Read the model definition and answer for the solid it produces. Units are mm, in the model's axes. Face numbers are marked on the shaded views. A direction names the side the tool comes from. Coordinates: 2 decimals unless noted, no trailing zeros. Write each loop counter-clockwise with the first axis right and the second up, starting at its lowest first coordinate (ties: lowest second). Pieces come first, ordered by that corner, then holes. Notation, with made-up numbers: (8, 43) -> (66, 43) arc R26 ccw to (66, 66) -> close; hole circle Ø5 at (-12, 46.5). An arc over 180 degrees is marked (long way). Write item = value, one per line. Start each with the question number.
1) A tool of negligible diameter and unlimited length cuts with its end or side. For the marked faces 1, 2, 3, 4 and 5, from which of +Z, -Z, +X, -X, +Y, -Y can it reach the whole face along a straight path? Write none if from no direction.
2) Section A-A (y = 0) is taken. Determine the outline of the cut face in (x, z).
3) Section B-B (z = -18) is taken. Determine the outline of the cut face in (x, y), plus the area to 3 significant figures.
4) Find the intervals of material crossed by line 1 along Z through (x, y) = (0, -0.5); line 2 along Y through (x, z) = (-7, 0); line 3 along Z through (x, y) = (-7.1, 0), in increasing order. Write a range as from..to.
5) For a pull along X with two mould halves and no side action, classify the marked faces 6, 7 and 8 as released by +X, released by -X, zero draft, split by the parting line, or undercut.
6) Section D-D (x = -1) is taken. Count the separate pieces of the cut face and the enclosed holes in it, plus the area to 3 significant figures.
7) Section C-C (z = -4) is taken. Determine the outline of the cut face in (x, y).
8) Flat-ended cylindrical pins translate along their axes: pin 1 Ø19 at (x, z) = (0, -18) entering from -Y; pin 2 Ø5 at (y, z) = (0, 0) entering from +X; pin 3 Ø3.5 at (y, z) = (0, -18) entering from -X; pin 4 Ø3 at (x, y) = (-1.5, -3) entering from +Z. Find the tip coordinate at first contact, or state that the pin passes through.
from build123d import *
from OCP.BRepFilletAPI import BRepFilletAPI_MakeChamfer

# Parameters (mm, degrees)
BOSS_EXTRUDE1_DEPTH     = 5
FILLET1_R               = 4
SKETCH2_R               = 8
BOSS_EXTRUDE2_DEPTH     = 0.5
SKETCH3_R               = 8
BOSS_EXTRUDE3_DEPTH     = 0.5
SKETCH4_R               = 8
BOSS_EXTRUDE4_DEPTH     = 0.5
CUT_EXTRUDE1_DEPTH      = 43.969085178
CUT_EXTRUDE1_DEPTH_BACK = 43.969085178
SKETCH5_R               = 6
CUT_EXTRUDE2_DEPTH      = 2
CHAMFER2_SIZE           = 1
CHAMFER2_SIZE2          = 1.732050808
CUT_EXTRUDE4_DEPTH      = 42.899788694
CUT_EXTRUDE4_DEPTH_BACK = 42.899788694
SKETCH9_R               = 1.5


with BuildPart() as part:
    # Sketch1 → Boss-Extrude1 (new, symmetric)
    with BuildSketch(Plane(origin=(0, 0, 0), x_dir=(1, 0, 0), z_dir=(0, 1, 0))):
        with BuildLine():
            Line((-10, 30.489995997), (-10, -2.679491924))
            Line((-10, -2.679491924), (-25.114071484, -6.729295173))
            ThreePointArc((-25.114071484, -6.729295173), (0, -26), (25.114071484, -6.729295173))
            Line((25.114071484, -6.729295173), (10, -2.679491924))
            Line((10, -2.679491924), (10, 30.489995997))
            ThreePointArc((10, 30.489995997), (0, 34), (-10, 30.489995997))
        make_face()
    extrude(amount=BOSS_EXTRUDE1_DEPTH, both=True)

    # Fillet1
    fillet1_edges = [part.edges().sort_by_distance(p)[0] for p in [
        (10, 0, -30.489995997),
        (10, 0, 2.679491924),
        (25.114071484, 0, 6.729295173),
        (-25.114071484, 0, 6.729295173),
        (-10, 0, 2.679491924),
        (-10, 0, -30.489995997),
    ]]
    fillet(fillet1_edges, radius=FILLET1_R)

    # Sketch2 → Boss-Extrude2 (add, symmetric)
    with BuildSketch(Plane(origin=(0, 0, 0), x_dir=(1, 0, 0), z_dir=(0, 1, 0))):
        with Locations((0, 18)):
            Circle(SKETCH2_R)
    extrude(amount=BOSS_EXTRUDE2_DEPTH, both=True)

    # Sketch3 → Boss-Extrude3 (add, symmetric)
    with BuildSketch(Plane(origin=(0, 5, 0), x_dir=(1, 0, 0), z_dir=(0, 1, 0))):
        with Locations(Location((0, 18, 0), (0, 0, 270))):
            Circle(SKETCH3_R)
    extrude(amount=BOSS_EXTRUDE3_DEPTH, both=True)

    # Sketch4 → Boss-Extrude4 (add, symmetric)
    with BuildSketch(Plane.XZ.offset(5)):
        with Locations(Location((0, 0, 0), (0, 0, 90))):
            Circle(SKETCH4_R)
    extrude(amount=BOSS_EXTRUDE4_DEPTH, both=True)

    # Sketch5 → Cut-Extrude1 (cut, two sides: drawn at the far end of the back side and taken through both)
    with BuildSketch(Plane(origin=(0, -5.5, 0), x_dir=(-1, 0, 0), z_dir=(0, -1, 0)).offset(-CUT_EXTRUDE1_DEPTH_BACK)):
        with Locations(Location((0, 0, 0), (0, 0, 90))):
            Circle(SKETCH5_R)
        with Locations(Location((0, 18, 0), (0, 0, 90))):
            Circle(SKETCH5_R)
    extrude(amount=CUT_EXTRUDE1_DEPTH + CUT_EXTRUDE1_DEPTH_BACK, mode=Mode.SUBTRACT)

    # Sketch6 → Cut-Extrude2 (cut)
    with BuildSketch(Plane(origin=(0, 5, 0), x_dir=(1, 0, 0), z_dir=(0, 1, 0))):
        with BuildLine():
            Line((12.188266684, -6.371664756), (20.119713435, -8.496889508))
            ThreePointArc((20.119713435, -8.496889508), (20.768948696, -9.043962883), (20.763662316, -9.892943304))
            ThreePointArc((20.763662316, -9.892943304), (0, -23), (-20.763662316, -9.892943304))
            ThreePointArc((-20.763662316, -9.892943304), (-20.768948696, -9.043962883), (-20.119713435, -8.496889508))
            Line((-20.119713435, -8.496889508), (-12.188266684, -6.371664756))
            ThreePointArc((-12.188266684, -6.371664756), (-11.342355786, -6.086056673), (-10.539679728, -5.695098402))
            ThreePointArc((-10.539679728, -5.695098402), (-9.810114884, -5.592432974), (-9.208235905, -6.017340901))
            ThreePointArc((-9.208235905, -6.017340901), (0, -11), (9.208235905, -6.017340901))
            ThreePointArc((9.208235905, -6.017340901), (9.810114884, -5.592432974), (10.539679728, -5.695098402))
            ThreePointArc((10.539679728, -5.695098402), (11.342355786, -6.086056673), (12.188266684, -6.371664756))
        make_face()
    cut_extrude2 = extrude(amount=-CUT_EXTRUDE2_DEPTH, mode=Mode.SUBTRACT)

    # Mirror7: Cut-Extrude2 across plane
    add(cut_extrude2.mirror(Plane.ZX), mode=Mode.SUBTRACT)

    # Chamfer2: one chamfer whose edges measure the first distance from different faces: ONE call of the kernel's chamfer builder (chamfer() names one face for all edges)
    chamfer2_edges_1 = [part.edges().sort_by_distance(p)[0] for p in [
        (9.810114884, -5, 5.592432974),
        (0, -5, 11),
        (-9.810114884, -5, 5.592432974),
        (-11.342355786, -5, 6.086056673),
        (-16.153990059, -5, 7.434277132),
        (-20.768948696, -5, 9.043962883),
        (0, -5, 23),
        (20.768948696, -5, 9.043962883),
        (16.153990059, -5, 7.434277132),
        (11.342355786, -5, 6.086056673),
    ]]
    chamfer2_side_1 = [part.faces().sort_by_distance(p)[0] for p in [
        (-9.233359985, -5, -14.391060437),
    ]]
    chamfer2_edges_2 = [part.edges().sort_by_distance(p)[0] for p in [
        (9.810114884, 5, 5.592432974),
    ]]
    chamfer2_side_2 = [part.faces().sort_by_distance(p)[0] for p in [
        (9.810114884, 4, 5.592432974),
    ]]
    chamfer2_edges_3 = [part.edges().sort_by_distance(p)[0] for p in [
        (0, 5, 11),
    ]]
    chamfer2_side_3 = [part.faces().sort_by_distance(p)[0] for p in [
        (0, 4, 11),
    ]]
    chamfer2_edges_4 = [part.edges().sort_by_distance(p)[0] for p in [
        (-9.810114884, 5, 5.592432974),
    ]]
    chamfer2_side_4 = [part.faces().sort_by_distance(p)[0] for p in [
        (-9.810114884, 4, 5.592432974),
    ]]
    chamfer2_edges_5 = [part.edges().sort_by_distance(p)[0] for p in [
        (-11.342355786, 5, 6.086056673),
    ]]
    chamfer2_side_5 = [part.faces().sort_by_distance(p)[0] for p in [
        (-11.342355786, 4, 6.086056673),
    ]]
    chamfer2_edges_6 = [part.edges().sort_by_distance(p)[0] for p in [
        (-16.153990059, 5, 7.434277132),
    ]]
    chamfer2_side_6 = [part.faces().sort_by_distance(p)[0] for p in [
        (-16.153990059, 4, 7.434277132),
    ]]
    chamfer2_edges_7 = [part.edges().sort_by_distance(p)[0] for p in [
        (-20.768948696, 5, 9.043962883),
    ]]
    chamfer2_side_7 = [part.faces().sort_by_distance(p)[0] for p in [
        (-20.768948696, 4, 9.043962883),
    ]]
    chamfer2_edges_8 = [part.edges().sort_by_distance(p)[0] for p in [
        (0, 5, 23),
    ]]
    chamfer2_side_8 = [part.faces().sort_by_distance(p)[0] for p in [
        (0, 4, 23),
    ]]
    chamfer2_edges_9 = [part.edges().sort_by_distance(p)[0] for p in [
        (20.768948696, 5, 9.043962883),
    ]]
    chamfer2_side_9 = [part.faces().sort_by_distance(p)[0] for p in [
        (20.768948696, 4, 9.043962883),
    ]]
    chamfer2_edges_10 = [part.edges().sort_by_distance(p)[0] for p in [
        (16.153990059, 5, 7.434277132),
    ]]
    chamfer2_side_10 = [part.faces().sort_by_distance(p)[0] for p in [
        (16.153990059, 4, 7.434277132),
    ]]
    chamfer2_edges_11 = [part.edges().sort_by_distance(p)[0] for p in [
        (11.342355786, 5, 6.086056673),
    ]]
    chamfer2_side_11 = [part.faces().sort_by_distance(p)[0] for p in [
        (11.342355786, 4, 6.086056673),
    ]]
    chamfer2 = BRepFilletAPI_MakeChamfer(part.part.solid().wrapped)
    for e in chamfer2_edges_1:
        chamfer2.Add(CHAMFER2_SIZE, CHAMFER2_SIZE2, e.wrapped, chamfer2_side_1[0].wrapped)  # the first distance lies on this face
    for e in chamfer2_edges_2:
        chamfer2.Add(CHAMFER2_SIZE, CHAMFER2_SIZE2, e.wrapped, chamfer2_side_2[0].wrapped)  # the first distance lies on this face
    for e in chamfer2_edges_3:
        chamfer2.Add(CHAMFER2_SIZE, CHAMFER2_SIZE2, e.wrapped, chamfer2_side_3[0].wrapped)  # the first distance lies on this face
    for e in chamfer2_edges_4:
        chamfer2.Add(CHAMFER2_SIZE, CHAMFER2_SIZE2, e.wrapped, chamfer2_side_4[0].wrapped)  # the first distance lies on this face
    for e in chamfer2_edges_5:
        chamfer2.Add(CHAMFER2_SIZE, CHAMFER2_SIZE2, e.wrapped, chamfer2_side_5[0].wrapped)  # the first distance lies on this face
    for e in chamfer2_edges_6:
        chamfer2.Add(CHAMFER2_SIZE, CHAMFER2_SIZE2, e.wrapped, chamfer2_side_6[0].wrapped)  # the first distance lies on this face
    for e in chamfer2_edges_7:
        chamfer2.Add(CHAMFER2_SIZE, CHAMFER2_SIZE2, e.wrapped, chamfer2_side_7[0].wrapped)  # the first distance lies on this face
    for e in chamfer2_edges_8:
        chamfer2.Add(CHAMFER2_SIZE, CHAMFER2_SIZE2, e.wrapped, chamfer2_side_8[0].wrapped)  # the first distance lies on this face
    for e in chamfer2_edges_9:
        chamfer2.Add(CHAMFER2_SIZE, CHAMFER2_SIZE2, e.wrapped, chamfer2_side_9[0].wrapped)  # the first distance lies on this face
    for e in chamfer2_edges_10:
        chamfer2.Add(CHAMFER2_SIZE, CHAMFER2_SIZE2, e.wrapped, chamfer2_side_10[0].wrapped)  # the first distance lies on this face
    for e in chamfer2_edges_11:
        chamfer2.Add(CHAMFER2_SIZE, CHAMFER2_SIZE2, e.wrapped, chamfer2_side_11[0].wrapped)  # the first distance lies on this face
    add(Compound.cast(chamfer2.Shape()), mode=Mode.REPLACE)

    # Sketch9 → Cut-Extrude4 (cut, two sides: drawn at the far end of the back side and taken through both)
    with BuildSketch(Plane(origin=(0, 0, 0), x_dir=(0, 0, -1), z_dir=(1, 0, 0)).offset(-CUT_EXTRUDE4_DEPTH_BACK)):
        Circle(SKETCH9_R)
        with Locations((18, 0)):
            Circle(SKETCH9_R)
    extrude(amount=CUT_EXTRUDE4_DEPTH + CUT_EXTRUDE4_DEPTH_BACK, mode=Mode.SUBTRACT)


solid = part.part
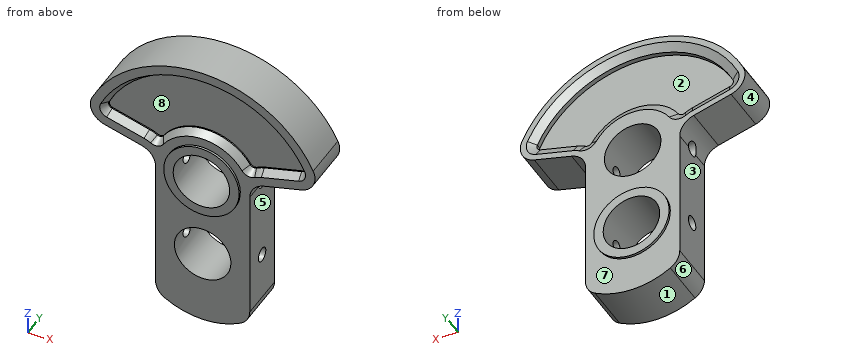
Answer key:
q1.face_1 = -Z, +Y, -Y
q1.face_2 = +Y
q1.face_3 = -Z, -X, +Y, -Y
q1.face_4 = -X, +Y, -Y
q1.face_5 = -Z, +X, +Y, -Y
q2.outline = (-23.47, 11.18) arc R4 ccw to (-20.9, 5.6) -> (-12.96, 3.47) arc R4 cw to (-10.47, 1.5) -> (-5.81, 1.5) arc R6 cw to (5.81, 1.5) -> (10.47, 1.5) arc R4 cw to (12.96, 3.47) -> (20.9, 5.6) arc R4 ccw to (23.47, 11.18) arc R26 ccw to start; (-10, -28.39) arc R4 ccw to (-8, -31.86) arc R16 ccw to (8, -31.86) arc R4 ccw to (10, -28.39) -> (10, -19.5) -> (5.81, -19.5) arc R6 cw to (-5.81, -19.5) -> (-10, -19.5) -> close; (-10, -16.5) -> (-5.81, -16.5) arc R6 cw to (5.81, -16.5) -> (10, -16.5) -> (10, -1.5) -> (5.81, -1.5) arc R6 cw to (-5.81, -1.5) -> (-10, -1.5) -> close
q3.outline = (-10, -5) -> (-6, -5) -> (-6, -1.5) -> (-10, -1.5) -> close; (-10, 1.5) -> (-6, 1.5) -> (-6, 5.5) -> (-8, 5.5) -> (-8, 5) -> (-10, 5) -> close; (6, -5) -> (10, -5) -> (10, -1.5) -> (6, -1.5) -> close; (6, 1.5) -> (10, 1.5) -> (10, 5) -> (8, 5) -> (8, 5.5) -> (6, 5.5) -> close
q3.area = 58.0 mm^2
q4.line_1 = -34..-24, -12..-6, 6..26
q4.line_2 = -5.5..-1.5, 1.5..5
q4.line_3 = -32.34..-19.5, -16.5..-1.5, 1.5..25.01
q5.face_6 = released by -X
q5.face_7 = zero draft
q5.face_8 = undercut
q6.separate_pieces = 3
q6.enclosed_holes = 0
q6.area = 315 mm^2
q7.outline = (-10, -5) -> (-6.93, -5) -> (-6.93, -5.5) -> (-4.47, -5.5) -> (-4.47, 5) -> (-10, 5) -> close; (4.47, -5.5) -> (6.93, -5.5) -> (6.93, -5) -> (10, -5) -> (10, 5) -> (4.47, 5) -> close
q8.pin_1 = -5
q8.pin_2 = 11.23
q8.pin_3 = -10
q8.pin_4 = 26
